Answer from the drawing. Dimensions are ordinates in mm from the lowest x, y and z of the part. A direction names the side the tool comes from. Give positions to 0.01 mm unless a question says otherwise; leave off trailing zeros. Write each loop counter-clockwise with the first axis right and the second up, starting at its lowest first coordinate (ties: lowest second). Pieces come first, ordered by that corner, then holes. Notation, with made-up numbers: (5, 68.5) -> (62, 68.5) arc R19 ccw to (62, 102.5) -> close; hole circle Ø8 at (-4.75, -0.5). An arc over 180 degrees is marked (long way). Use a Markdown table: item, result. Add a question column.
Q1. Section A-A, the plane x = 140 is taken. Give the vertices of the cut face in (y, z), plus the area to 3 significant figures.
Q2. Consider line 1 (Z direction, x = 140, y = 18.5); line 2 (X direction, y = 39, z = 165); line 3 (X direction, y = 47.5, z = 40). Determine where each line is inside the solid, lowest interval first.
Q3. Section B-B, the plane z = 165 is taken. Give the vertices of the cut face in (x, y), plus the area to 3 significant figures.
Q4. For the marked faces 1, 2 and 3, determine the directions among +Z, -Z, +X, -X, +Y, -Y from which every point of the face is accessible in a straight line to the end or side of a thin tool.
Q5. For a pull along X with two mould halves and no side action, classify the marked faces 4, 5, 6 and 7 as pulls with the +X half, pulls with the -X half, needs draft (parallel to the pull), parting line crosses it, or undercut.
Q6. Each of these flat-tipped pins is pushed along its axis until it touches: pin 1 Ø10 at (x, y) = (84, 25.5) entering from -Z; pin 2 Ø1 at (y, z) = (8, 21) entering from +X. Where does it stop, or does it pass through?
Q7. Section C-C, the plane y = 7.5 is taken. Give the vertices of the cut face in (x, z), plus the area to 3 significant figures.
Q8. Section D-D, the plane x = 240 is taken. Give the vertices of the cut face in (y, z).
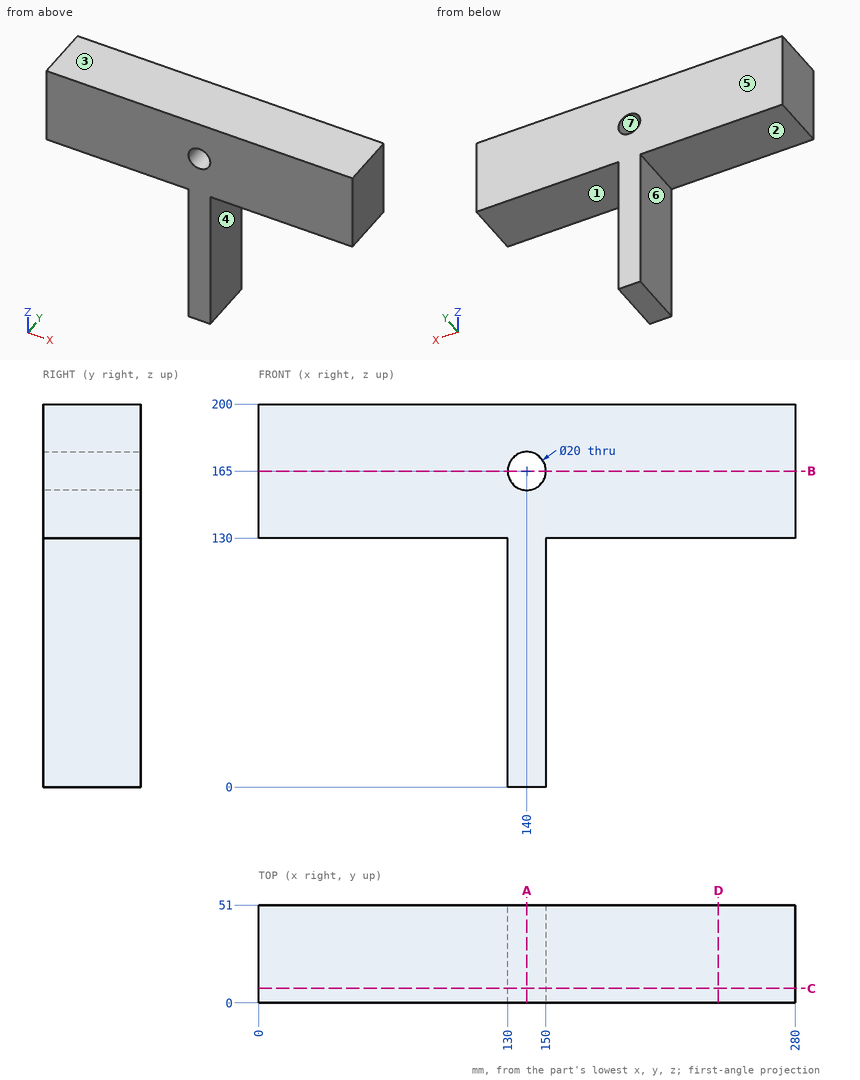
Result set:
| question | item | result |
|---|---|---|
| 1 | outline | (0, 0) -> (51, 0) -> (51, 155) -> (0, 155) -> close; (0, 175) -> (51, 175) -> (51, 200) -> (0, 200) -> close |
| 1 | area | 9,180 mm2 |
| 2 | line 1 | z = 0 to 155, 175 to 200 |
| 2 | line 2 | x = 0 to 130, 150 to 280 |
| 2 | line 3 | x = 130 to 150 |
| 3 | outline | (0, 0) -> (130, 0) -> (130, 51) -> (0, 51) -> close; (150, 0) -> (280, 0) -> (280, 51) -> (150, 51) -> close |
| 3 | area | 13,300 mm2 |
| 4 | face 1 | -Z, +X, +Y, -Y |
| 4 | face 2 | -Z, -X, +Y, -Y |
| 4 | face 3 | +Z, +X, -X, +Y, -Y |
| 5 | face 4 | pulls with the +X half |
| 5 | face 5 | needs draft |
| 5 | face 6 | pulls with the -X half |
| 5 | face 7 | undercut |
| 6 | pin 1 | stops at z = 130 |
| 6 | pin 2 | stops at x = 150 |
| 7 | outline | (0, 130) -> (130, 130) -> (130, 0) -> (150, 0) -> (150, 130) -> (280, 130) -> (280, 200) -> (0, 200) -> close; hole circle Ø20 at (140, 165) |
| 7 | area | 21,900 mm2 |
| 8 | outline | (0, 130) -> (51, 130) -> (51, 200) -> (0, 200) -> close |
